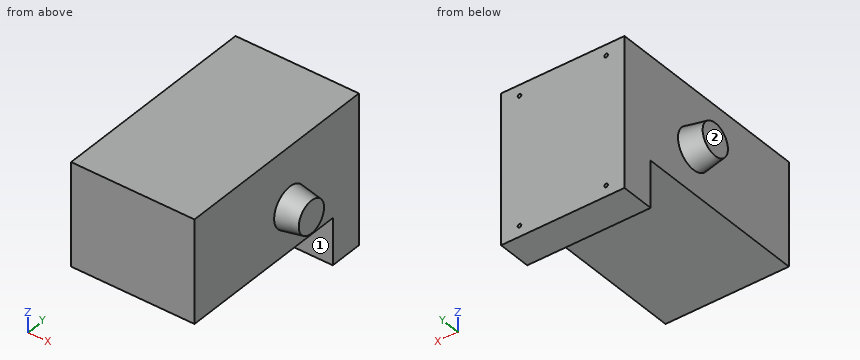
from build123d import *

# Parameters (mm, degrees)
SKETCH_1_W                  = 114
SKETCH_1_H                  = 95
EXTRUDE_1_DEPTH             = 164
SKETCH_2_W                  = 114
SKETCH_2_H                  = 138
EXTRUDE_2_DEPTH             = 31
PATTERN_LINEAR_1_COUNT      = 2
PATTERN_LINEAR_1_PITCH      = 118
PATTERN_LINEAR_1_COUNT_DIR2 = 2
PATTERN_LINEAR_1_PITCH_DIR2 = 80
SKETCH_6_R                  = 15
EXTRUDE_3_DEPTH             = 20
DRAFT_1_ANGLE               = 10


with BuildPart() as part:
    # Sketch 1 → Extrude 1 (new body)
    with BuildSketch(Plane(origin=(0, 0, 0), x_dir=(1, 0, 0), z_dir=(0, 1, 0))):
        Rectangle(SKETCH_1_W, SKETCH_1_H)
    extrude(amount=EXTRUDE_1_DEPTH)

    # Sketch 2 → Extrude 2 (add)
    with BuildSketch(Plane(origin=(0, 164, 0), x_dir=(1, 0, 0), z_dir=(0, 1, 0))):
        with Locations((0, 21.5)):
            Rectangle(SKETCH_2_W, SKETCH_2_H)
    extrude(amount=EXTRUDE_2_DEPTH)

    # Sketch 5 → Hole Wizard M4 _1 (revolve, cut)
    with BuildSketch(Plane(origin=(-40, 195, 37.5), x_dir=(0, 0, 1), z_dir=(1, 0, 0))):
        Polygon((0, 0), (0, 8.991420021), (1.65, 8), (1.65, 0), align=None)
    hole_wizard_m4_1 = revolve(axis=Axis((-40, 201.35, 37.5), (0, -1, 0)), mode=Mode.SUBTRACT)

    # Pattern Linear 1: Hole Wizard M4 _1 2 × 2
    with Locations(*[(j * PATTERN_LINEAR_1_PITCH_DIR2, 0, -i * PATTERN_LINEAR_1_PITCH) for i in range(PATTERN_LINEAR_1_COUNT) for j in range(PATTERN_LINEAR_1_COUNT_DIR2) if (i, j) != (0, 0)]):
        add(hole_wizard_m4_1, mode=Mode.SUBTRACT)

    # Sketch 6 → Extrude 3 (add)
    with BuildSketch(Plane(origin=(57, 0, 0), x_dir=(0, 0, -1), z_dir=(1, 0, 0))):
        with Locations(Location((7.5, 113, 0), (0, 0, 180))):
            Circle(SKETCH_6_R)
    extrude(amount=EXTRUDE_3_DEPTH)

    # Draft 1
    draft_1_faces = [part.faces().sort_by_distance(p)[0] for p in [
        (67, 113, -22.5),
    ]]
    draft(draft_1_faces, Plane(origin=(77, 113, -7.5), x_dir=(0, 0, 1), z_dir=(1, 0, 0)), DRAFT_1_ANGLE)

    # Mirror 1: part across plane


with BuildPart() as part_1:
    add(part.part)
    add(part.part.mirror(Plane(origin=(0, 0, 0), x_dir=(0, 0, 1), z_dir=(1, 0, 0))))


solid = part_1.part
Read the model definition and answer for the solid it produces. Units are mm, in the model's axes. Face numbers are marked on the shaded views. A direction names the side the tool comes from. Give positions to 0.01 mm unless a question says otherwise; leave off trailing zeros. Write each loop counter-clockwise with the first axis right and the second up, starting at its lowest first coordinate (ties: lowest second). Pieces come first, ordered by that corner, then holes. Notation, with made-up numbers: (28, 1.5) - (42, 1.5) arc R15 cw to (42, 14.5) - close; hole circle Ø11 at (61.25, 38). An arc over 180 degrees is marked (long way). Return JSON: item names as keys, results as strings.
Q1. Given P1, Ø2.5, axis at x = 40, z = 37.5, coming from the +Y side; P2, Ø2, axis at x = -6, z = 13.5, coming from the -Y side; P3, Ø12, axis at x = -54, y = 62.5, coming from the -Z side; P4, Ø2, axis at y = 173, z = 11, coming from the -X side, each flat-ended and moving along its own axis, determine where each tip first touches the part or whether it passes through.
Reply:
{"P1": "y = 186.76", "P2": "y = 0", "P3": "z = -47.5", "P4": "x = -57"}
Q2. Consider line 1 along Z through (x, y) = (40, 192.25); line 2 along X through (y, z) = (189.25, -80.5); line 3 along X through (y, z) = (122, 23). Determine where each line is inside the solid, lowest interval first. Write a range as [from, to].
Reply:
{"line 1": "[-90.5, -82.15], [-78.85, 35.85], [39.15, 47.5]", "line 2": "[-57, -41.65], [-38.35, 38.35], [41.65, 57]", "line 3": "[-57, 57]"}
Q3. A cutting plane is placed at B-B, the plane x = -8. Determine the outline of the cut face in (y, z).
Reply:
{"outline": "(0, -47.5) - (164, -47.5) - (164, -90.5) - (195, -90.5) - (195, 47.5) - (0, 47.5) - close"}
Q4. A cutting plane is placed at A-A, the plane z = -7.5. Determine the outline of the cut face in (x, y).
Reply:
{"outline": "(-77, 98) - (-57, 94.47) - (-57, 0) - (57, 0) - (57, 94.47) - (77, 98) - (77, 128) - (57, 131.53) - (57, 195) - (-57, 195) - (-57, 131.53) - (-77, 128) - close"}
Q5. A cutting plane is placed at C-C, the plane z = -63. Determine the outline of the cut face in (x, y).
Reply:
{"outline": "(-57, 164) - (57, 164) - (57, 195) - (-57, 195) - close"}
Q6. For the marked faces 1 and 2, determine the directions among +Z, -Z, +X, -X, +Y, -Y from which every point of the face is accessible in a straight line to the end or side of a thin tool.
Reply:
{"face 1": "-Z, +X, -X, -Y", "face 2": "+Z, -Z, -X, +Y, -Y"}
Q7. A cutting plane is placed at D-D, the plane z = -35. Determine the outline of the cut face in (x, y).
Reply:
{"outline": "(-57, 0) - (57, 0) - (57, 195) - (-57, 195) - close"}
